```python
from build123d import *

# Parameters (mm, degrees)
SKETCH_1_R      = 1.5
SKETCH_1_R_2    = 9
EXTRUDE_1_DEPTH = 6


with BuildPart() as part:
    # 草图1 → 凸台-拉伸1 (new body)
    with BuildSketch(Plane(origin=(0, 0, 0), x_dir=(-1, 0, 0), z_dir=(0, 0, -1))):
        with BuildLine():
            Line((32.955703333, 66.620894067), (30.80974204, 91.149343878))
            ThreePointArc((30.80974204, 91.149343878), (13.132902588, 106.651516018), (-3.125567827, 89.667696251))
            Line((-3.125567827, 89.667696251), (-3.125567827, 46.910336938))
            ThreePointArc((-3.125567827, 46.910336938), (-3.35392923, 45.762286641), (-4.004247484, 44.789016595))
            Line((-4.004247484, 44.789016595), (-6.246888171, 42.546375908))
            ThreePointArc((-6.246888171, 42.546375908), (-6.897206425, 41.573105861), (-7.125567827, 40.425055564))
            Line((-7.125567827, 40.425055564), (-7.125567827, 18.910336938))
            ThreePointArc((-7.125567827, 18.910336938), (-6.897206425, 17.762286641), (-6.246888171, 16.789016595))
            Line((-6.246888171, 16.789016595), (-4.004247484, 14.546375908))
            ThreePointArc((-4.004247484, 14.546375908), (-3.35392923, 13.573105861), (-3.125567827, 12.425055564))
            Line((-3.125567827, 12.425055564), (-3.125567827, 10.910336938))
            ThreePointArc((-3.125567827, 10.910336938), (-3.35392923, 9.762286641), (-4.004247484, 8.789016595))
            Line((-4.004247484, 8.789016595), (-6.246888171, 6.546375908))
            ThreePointArc((-6.246888171, 6.546375908), (-6.897206425, 5.573105861), (-7.125567827, 4.425055564))
            Line((-7.125567827, 4.425055564), (-7.125567827, -13.089663062))
            ThreePointArc((-7.125567827, -13.089663062), (-6.897206425, -14.237713359), (-6.246888171, -15.210983405))
            Line((-6.246888171, -15.210983405), (-4.004247484, -17.453624092))
            ThreePointArc((-4.004247484, -17.453624092), (-3.35392923, -18.426894139), (-3.125567827, -19.574944436))
            Line((-3.125567827, -19.574944436), (-3.125567827, -29.86687526))
            ThreePointArc((-3.125567827, -29.86687526), (-3.090102825, -30.326801608), (-2.98454633, -30.775853763))
            Line((-2.98454633, -30.775853763), (4.301916011, -53.693710595))
            ThreePointArc((4.301916011, -53.693710595), (19.95472423, -60.194746986), (23.749643638, -43.67589515))
            ThreePointArc((23.749643638, -43.67589515), (23.452277042, -43.108350682), (23.349643638, -42.47589515))
            Line((23.349643638, -42.47589515), (23.349643638, -4.902719504))
            ThreePointArc((23.349643638, -4.902719504), (23.040438051, -3.834443205), (22.208429387, -3.096483906))
            ThreePointArc((22.208429387, -3.096483906), (18.784786633, 2.32222289), (22.208429387, 7.740929686))
            ThreePointArc((22.208429387, 7.740929686), (23.040438051, 8.478888986), (23.349643638, 9.547165285))
            Line((23.349643638, 9.547165285), (23.349643638, 12.31993364))
            ThreePointArc((23.349643638, 12.31993364), (22.903935561, 13.578574422), (21.765467019, 14.276228841))
            Line((21.765467019, 14.276228841), (19.563528405, 14.744265342))
            ThreePointArc((19.563528405, 14.744265342), (18.30201065, 15.611282474), (18.023056585, 17.116383925))
            Line((18.023056585, 17.116383925), (21.012916503, 31.182568919))
            ThreePointArc((21.012916503, 31.182568919), (21.710570922, 32.32103746), (22.969211704, 32.766745537))
            Line((22.969211704, 32.766745537), (28.907131585, 32.766745537))
            ThreePointArc((28.907131585, 32.766745537), (30.321345148, 33.352531975), (30.907131585, 34.766745537))
            Line((30.907131585, 34.766745537), (30.907131585, 62.915918647))
            ThreePointArc((30.907131585, 62.915918647), (31.129655766, 63.83274999), (31.747711296, 64.545564189))
            ThreePointArc((31.747711296, 64.545564189), (31.948812633, 64.689858135), (32.148749116, 64.835761848))
            ThreePointArc((32.148749116, 64.835761848), (32.785761883, 65.622760099), (32.955703333, 66.620894067))
        make_face()
        with Locations((13.874432173, 100.667696251)):
            Circle(SKETCH_1_R, mode=Mode.SUBTRACT)
        with Locations((4.348152731, 95.167696251)):
            Circle(SKETCH_1_R, mode=Mode.SUBTRACT)
        with Locations((4.348152731, 84.167696251)):
            Circle(SKETCH_1_R, mode=Mode.SUBTRACT)
        with Locations((13.874432173, 78.667696251)):
            Circle(SKETCH_1_R, mode=Mode.SUBTRACT)
        with Locations((23.400711614, 84.167696251)):
            Circle(SKETCH_1_R, mode=Mode.SUBTRACT)
        with Locations((12.874432173, -22.332303749)):
            Circle(SKETCH_1_R, mode=Mode.SUBTRACT)
        with Locations((2.874432173, -14.332303749)):
            Circle(SKETCH_1_R, mode=Mode.SUBTRACT)
        with Locations((12.874432173, -34.332303749)):
            Circle(SKETCH_1_R, mode=Mode.SUBTRACT)
        with Locations((2.874432173, -34.332303749)):
            Circle(SKETCH_1_R, mode=Mode.SUBTRACT)
        with Locations((14.874432173, -50.332303749)):
            Circle(SKETCH_1_R_2, mode=Mode.SUBTRACT)
        with Locations((23.400711614, 95.167696251)):
            Circle(SKETCH_1_R, mode=Mode.SUBTRACT)
        with BuildLine():
            Line((-2.107533838, 35.667696251), (-1.143601816, 35.667696251))
            ThreePointArc((-1.143601816, 35.667696251), (-0.735353525, 35.754825322), (-0.398245823, 36.001029585))
            ThreePointArc((-0.398245823, 36.001029585), (0.327985563, 36.021249642), (0.307765506, 35.295018255))
            ThreePointArc((0.307765506, 35.295018255), (0.061561244, 34.957910553), (-0.025567827, 34.549662262))
            Line((-0.025567827, 34.549662262), (-0.025567827, 24.78573024))
            ThreePointArc((-0.025567827, 24.78573024), (0.061561244, 24.377481949), (0.307765506, 24.040374247))
            ThreePointArc((0.307765506, 24.040374247), (0.327985563, 23.314142861), (-0.398245823, 23.334362918))
            ThreePointArc((-0.398245823, 23.334362918), (-0.735353525, 23.58056718), (-1.143601816, 23.667696251))
            Line((-1.143601816, 23.667696251), (-2.107533838, 23.667696251))
            ThreePointArc((-2.107533838, 23.667696251), (-2.515782129, 23.58056718), (-2.852889831, 23.334362918))
            ThreePointArc((-2.852889831, 23.334362918), (-3.579121218, 23.314142861), (-3.558901161, 24.040374247))
            ThreePointArc((-3.558901161, 24.040374247), (-3.312696898, 24.377481949), (-3.225567827, 24.78573024))
            Line((-3.225567827, 24.78573024), (-3.225567827, 34.549662262))
            ThreePointArc((-3.225567827, 34.549662262), (-3.312696898, 34.957910553), (-3.558901161, 35.295018255))
            ThreePointArc((-3.558901161, 35.295018255), (-3.579121218, 36.021249642), (-2.852889831, 36.001029585))
            ThreePointArc((-2.852889831, 36.001029585), (-2.515782129, 35.754825322), (-2.107533838, 35.667696251))
        make_face(mode=Mode.SUBTRACT)
        with BuildLine():
            Line((10.874432173, 95.412258898), (10.874432173, 96.667696251))
            ThreePointArc((10.874432173, 96.667696251), (11.167325392, 97.374803032), (11.874432173, 97.667696251))
            Line((11.874432173, 97.667696251), (15.874432173, 97.667696251))
            ThreePointArc((15.874432173, 97.667696251), (16.581538954, 97.374803032), (16.874432173, 96.667696251))
            Line((16.874432173, 96.667696251), (16.874432173, 95.412258898))
            ThreePointArc((16.874432173, 95.412258898), (16.988026912, 94.949348848), (17.303003601, 94.591607091))
            ThreePointArc((17.303003601, 94.591607091), (13.874432173, 83.667696251), (10.445860744, 94.591607091))
            ThreePointArc((10.445860744, 94.591607091), (10.760837433, 94.949348848), (10.874432173, 95.412258898))
        make_face(mode=Mode.SUBTRACT)
        with BuildLine():
            Line((11.374432172, 65.152523811), (16.374432175, 62.265772463))
            ThreePointArc((16.374432175, 62.265772463), (17.874432175, 59.667696252), (16.374432175, 57.06962004))
            Line((16.374432175, 57.06962004), (11.374432172, 54.182868693))
            ThreePointArc((11.374432172, 54.182868693), (8.374432172, 54.182868693), (6.874432172, 56.780944904))
            Line((6.874432172, 56.780944904), (6.874432172, 62.5544476))
            ThreePointArc((6.874432172, 62.5544476), (8.374432172, 65.152523811), (11.374432172, 65.152523811))
        make_face(mode=Mode.SUBTRACT)
        with BuildLine():
            Line((6.874432172, 8.780944893), (6.874432172, 14.554447588))
            ThreePointArc((6.874432172, 14.554447588), (8.374432172, 17.1525238), (11.374432172, 17.1525238))
            Line((11.374432172, 17.1525238), (16.374432175, 14.265772452))
            ThreePointArc((16.374432175, 14.265772452), (17.874432175, 11.66769624), (16.374432175, 9.069620029))
            Line((16.374432175, 9.069620029), (11.374432172, 6.182868681))
            ThreePointArc((11.374432172, 6.182868681), (8.374432172, 6.182868681), (6.874432172, 8.780944893))
        make_face(mode=Mode.SUBTRACT)
        with BuildLine():
            Line((13.874432173, -4.373755645), (9.874432172, -2.064354567))
            ThreePointArc((9.874432172, -2.064354567), (8.874432172, -0.33230376), (9.874432172, 1.399747048))
            Line((9.874432172, 1.399747048), (13.874432173, 3.709148125))
            ThreePointArc((13.874432173, 3.709148125), (15.874432173, 3.709148125), (16.874432173, 1.977097318))
            Line((16.874432173, 1.977097318), (16.874432173, -2.641704837))
            ThreePointArc((16.874432173, -2.641704837), (15.874432173, -4.373755645), (13.874432173, -4.373755645))
        make_face(mode=Mode.SUBTRACT)
        with BuildLine():
            Line((6.874432172, -15.219055113), (6.874432172, -9.445552417))
            ThreePointArc((6.874432172, -9.445552417), (8.374432172, -6.847476206), (11.374432172, -6.847476206))
            Line((11.374432172, -6.847476206), (16.374432175, -9.734227554))
            ThreePointArc((16.374432175, -9.734227554), (17.874432175, -12.332303765), (16.374432175, -14.930379977))
            Line((16.374432175, -14.930379977), (11.374432172, -17.817131325))
            ThreePointArc((11.374432172, -17.817131325), (8.374432172, -17.817131325), (6.874432172, -15.219055113))
        make_face(mode=Mode.SUBTRACT)
        with BuildLine():
            Line((9.874432172, 25.399747048), (13.874432173, 27.709148125))
            ThreePointArc((13.874432173, 27.709148125), (15.874432173, 27.709148125), (16.874432173, 25.977097318))
            Line((16.874432173, 25.977097318), (16.874432173, 21.358295163))
            ThreePointArc((16.874432173, 21.358295163), (15.874432173, 19.626244355), (13.874432173, 19.626244355))
            Line((13.874432173, 19.626244355), (9.874432172, 21.935645433))
            ThreePointArc((9.874432172, 21.935645433), (8.874432172, 23.66769624), (9.874432172, 25.399747048))
        make_face(mode=Mode.SUBTRACT)
        with BuildLine():
            Line((20.874432175, 50.554447597), (20.874432175, 44.780944901))
            ThreePointArc((20.874432175, 44.780944901), (19.374432175, 42.18286869), (16.374432175, 42.18286869))
            Line((16.374432175, 42.18286869), (11.374432172, 45.069620038))
            ThreePointArc((11.374432172, 45.069620038), (9.874432172, 47.667696249), (11.374432172, 50.26577246))
            Line((11.374432172, 50.26577246), (16.374432175, 53.152523808))
            ThreePointArc((16.374432175, 53.152523808), (19.374432175, 53.152523808), (20.874432175, 50.554447597))
        make_face(mode=Mode.SUBTRACT)
        with BuildLine():
            Line((-3.225567827, -9.21426976), (-3.225567827, 0.549662262))
            ThreePointArc((-3.225567827, 0.549662262), (-3.312696898, 0.957910553), (-3.558901161, 1.295018255))
            ThreePointArc((-3.558901161, 1.295018255), (-3.579121218, 2.021249642), (-2.852889831, 2.001029585))
            ThreePointArc((-2.852889831, 2.001029585), (-2.515782129, 1.754825322), (-2.107533838, 1.667696251))
            Line((-2.107533838, 1.667696251), (-1.143601816, 1.667696251))
            ThreePointArc((-1.143601816, 1.667696251), (-0.735353525, 1.754825322), (-0.398245823, 2.001029585))
            ThreePointArc((-0.398245823, 2.001029585), (0.327985563, 2.021249642), (0.307765506, 1.295018255))
            ThreePointArc((0.307765506, 1.295018255), (0.061561244, 0.957910553), (-0.025567827, 0.549662262))
            Line((-0.025567827, 0.549662262), (-0.025567827, -9.21426976))
            ThreePointArc((-0.025567827, -9.21426976), (0.061561244, -9.622518051), (0.307765506, -9.959625753))
            ThreePointArc((0.307765506, -9.959625753), (0.327985563, -10.685857139), (-0.398245823, -10.665637082))
            ThreePointArc((-0.398245823, -10.665637082), (-0.735353525, -10.41943282), (-1.143601816, -10.332303749))
            Line((-1.143601816, -10.332303749), (-2.107533838, -10.332303749))
            ThreePointArc((-2.107533838, -10.332303749), (-2.515782129, -10.41943282), (-2.852889831, -10.665637082))
            ThreePointArc((-2.852889831, -10.665637082), (-3.579121218, -10.685857139), (-3.558901161, -9.959625753))
            ThreePointArc((-3.558901161, -9.959625753), (-3.312696898, -9.622518051), (-3.225567827, -9.21426976))
        make_face(mode=Mode.SUBTRACT)
    extrude(amount=-EXTRUDE_1_DEPTH)


solid = part.part
```
Here's how the part is built. I have some questions about the finished solid (model axes, mm). A direction names the side the tool comes from. Round coordinates to 2 decimals unless told otherwise and drop trailing zeros. Order: outer loops, then holes, each group sorted by start corner. A loop starts at its lowest first (then second) coordinate and runs counter-clockwise, first axis right, second up. Notation, with made-up numbers: M 35.25,-38 L 67.25,-38 A26 cw 67.25,0 Z; hole C 72,52.5 d2. An arc over 180 degrees is marked long. Use CSV: the item, a comma, the result in double quotes.
1) I want a section at A-A (y = 71). List the corners of the cut face in (x, z) for me.
Taken from the geometry:
outline,"M -32.57,0 L 3.13,0 L 3.13,6 L -32.57,6 Z"
2) I need wall thicknesses on line 1 along X through (y, z) = (25.5, 4.9); line 2 along X through (y, z) = (1.5, 4.4); line 3 along Y through (x, z) = (-23, 2.75). Which ranges of each line are inside material? Lowest first, please. Write a range as [from, to].
Taken from the geometry:
line 1,"[-19.81, -16.87], [-10.05, 0.03], [3.23, 7.13]"
line 2,"[-18.84, -16.87], [-10.05, -0.45], [3.7, 7.13]"
line 3,"[-57.89, -54.2], [-46.46, -3.77], [8.42, 13.45], [32.77, 82.72], [85.61, 93.72], [96.61, 104.01]"
3) I'm going to push flat-ended pins straight in: P1, Ø2.5, axis at x = -12.87, y = -22.33, coming from the -Z side; P2, Ø2, axis at x = -8, z = 5.5, coming from the -Y side; P3, Ø3, axis at y = -20, z = 2, coming from the -X side; P4, Ø1.4, axis at y = 96, z = 2, coming from the +X side. Where does each tip first touch, or does it pass through?
Taken from the geometry:
P1,"through"
P2,"y = -59.74"
P3,"x = -23.35"
P4,"x = 2.17"
4) If we mould it in two halves opening along X, with no side actions, what happens to faces 1 (the flat face through (-0.608, -42.074, 2.958)), 2 (the cylindrical face through (-8.337, -6.87, 2.958))? For each: pulls with the +X half, pulls with the -X half, needs draft (parallel to the pull), parting line crosses it, or undercut.
Taken from the geometry:
face 1,"pulls with the +X half"
face 2,"undercut"
5) On a 3-axis mill with a long thin cutter (end or side, diameter ignored), from which of +Z, -Z, +X, -X, +Y, -Y can I reach the whole of each face in a straight line? I mean faces 3 (the flat face through (3.126, 69, 3)), 4 (the flat face through (-13.84, 51.69, 2.96)). Say none if no direction works.
Taken from the geometry:
face 3,"+Z, -Z, +X, +Y"
face 4,"+Z, -Z"
6) I want a section at B-B (z = 2.25). Count the separate pieces of the cut face and the enclosed holes in it, then the cut area to 3 significant figures.
Taken from the geometry:
separate pieces,"1"
enclosed holes,"20"
area,"3,850 mm^2"
